```python
from build123d import *

# Parameters (mm, degrees)
F0_R     = 4.55
F0_R_2   = 6.95
F0_R_3   = 0.65
F1_DEPTH = 1.6


with BuildPart() as f1:
    # F0 (on Right) → F1 (new body)
    with BuildSketch(Plane.YZ):
        Polygon((5.01199, -29.453935), (14.8, -20.449221), (14.8, 11.000779), (27.1, 11.000779), (27.1, 13.000779), (32.4, 13.000779), (32.4, 21.460779), (25.571501, 23.000779), (8.571501, 23.000779), (-19.723812, 10.790342), (-8.867455, -14.367152), align=None)
        with Locations((5.75, -15.934274)):
            Circle(F0_R, mode=Mode.SUBTRACT)
        Circle(F0_R_2, mode=Mode.SUBTRACT)
        with Locations((9.462554, 21.492073)):
            Circle(F0_R_3, mode=Mode.SUBTRACT)
        with Locations((13.662554, 21.43904)):
            Circle(F0_R_3, mode=Mode.SUBTRACT)
    extrude(amount=F1_DEPTH)


solid = f1.part
```
Check sheet for the modelled part. Datum: model origin and axes. Units: mm. A direction names the side the tool comes from. Give positions to 0.01 mm unless a question says otherwise; leave off trailing zeros. Order: outer loops, then holes, each group sorted by start corner. A loop starts at its lowest first (then second) coordinate and runs counter-clockwise, first axis right, second up. Notation, with made-up numbers: (-36, 18.25) -> (-31, 18.25) arc R25 cw to (-31, 39.25) -> close; hole circle Ø11 at (77, 27.25). An arc over 180 degrees is marked (long way). Use CSV: the item, a comma, the result in double quotes. Start each with the question number.
1) Set-up check for faces 1 (the face through (0.789, 13.013, 21.468)), 2 (the face through (1, 30, 13.001)): record each of +Z, -Z, +X, -X, +Y, -Y from which the full face is reachable in a straight line by a thin tool's end or side.
2) Sectioned sample at D-D, the plane x = 1.1. Record the boundary of the cut face in (y, z).
3) Go/stop test with a flat-tipped pin: P1, Ø0.5, axis at x = 1, y = 20.5, coming from the -Z side. Record where the tip stops, or that it passes through.
4) Sectioned sample at C-C, the plane y = 0. Record the boundary of the cut face in (x, z).
5) Material ranges on line 1 (Y direction, x = 1.4, z = -15); line 2 (Z direction, x = 0.6, y = 0.5); line 3 (Y direction, x = 1.5, z = 5.5), recorded low to high. Write a range as from..to.
6) Sectioned sample at B-B, the plane y = 5.75. Record the boundary of the cut face in (x, z), plus the area to 3 significant figures.
7) Sectioned sample at A-A, the plane z = -17. Record the boundary of the cut face in (x, y), plus the area to 3 significant figures.
8) Mould release check, pull along Y, two halves, no side actions. Record for faces 3 (the face through (0.789, -14.372, -1.612)), 4 (the face through (1, 27.1, 12)), 5 (the face through (0.79, 8.98, 21.93)): released by +Y, released by -Y, zero draft, split by the parting line, or undercut.
Recorded:
1,face 1,"+X, -X"
1,face 2,"-Z, +X, -X, +Y"
2,outline,"(-19.72, 10.79) -> (-8.87, -14.37) -> (5.01, -29.45) -> (14.8, -20.45) -> (14.8, 11) -> (27.1, 11) -> (27.1, 13) -> (32.4, 13) -> (32.4, 21.46) -> (25.57, 23) -> (8.57, 23) -> close; hole circle Ø13.9 at (0, 0); hole circle Ø9.1 at (5.75, -15.93); hole circle Ø1.3 at (9.46, 21.49); hole circle Ø1.3 at (13.66, 21.44)"
3,P1,"z = 11"
4,outline,"(0, -24.01) -> (1.6, -24.01) -> (1.6, -6.95) -> (0, -6.95) -> close; (0, 6.95) -> (1.6, 6.95) -> (1.6, 19.3) -> (0, 19.3) -> close"
5,line 1,"-8.29..1.3, 10.2..14.8"
5,line 2,"-24.55..-6.93, 6.93..19.52"
5,line 3,"-17.44..-4.25, 4.25..14.8"
6,outline,"(0, -28.77) -> (1.6, -28.77) -> (1.6, -20.48) -> (0, -20.48) -> close; (0, -11.38) -> (1.6, -11.38) -> (1.6, -3.9) -> (0, -3.9) -> close; (0, 3.9) -> (1.6, 3.9) -> (1.6, 21.78) -> (0, 21.78) -> close"
6,area,"53.8 mm2"
7,outline,"(0, -6.45) -> (1.6, -6.45) -> (1.6, 1.33) -> (0, 1.33) -> close; (0, 10.17) -> (1.6, 10.17) -> (1.6, 14.8) -> (0, 14.8) -> close"
7,area,"19.8 mm2"
8,face 3,"released by -Y"
8,face 4,"released by +Y"
8,face 5,"undercut"
